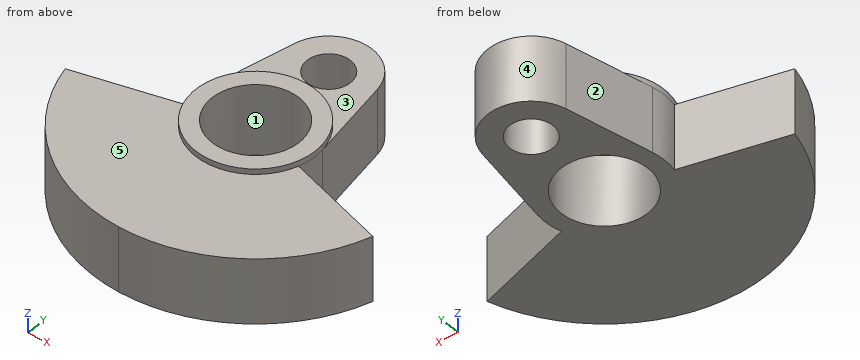
```python
from build123d import *
from build123d.topology import SkipClean

# Parameters (mm, degrees)
SKETCH1_R           = 2
SKETCH1_R_2         = 4
BOSS_EXTRUDE1_DEPTH = 6
BOSS_EXTRUDE2_START = -6
BOSS_EXTRUDE2_DEPTH = 6
SKETCH3_R           = 5.5
SKETCH3_R_2         = 4
BOSS_EXTRUDE4_DEPTH = 0.5


with BuildPart() as part:
    # Sketch1 → Boss-Extrude1 (new body)
    with BuildSketch(Plane.XY):
        with BuildLine():
            Line((-5.402455316, -6.96875), (-3.929058411, 0.75))
            ThreePointArc((-3.929058411, 0.75), (0, 4), (3.929058411, 0.75))
            Line((3.929058411, 0.75), (5.402455316, -6.96875))
            ThreePointArc((5.402455316, -6.96875), (0, -13.5), (-5.402455316, -6.96875))
        make_face()
        Circle(SKETCH1_R, mode=Mode.SUBTRACT)
        with Locations((0, -8)):
            Circle(SKETCH1_R_2, mode=Mode.SUBTRACT)
    extrude(amount=BOSS_EXTRUDE1_DEPTH)

    # Sketch2 → Boss-Extrude2 (add)
    with BuildSketch(Plane.XY.offset(6).offset(BOSS_EXTRUDE2_START)):
        with BuildLine():
            Line((0, -13.5), (0, -23))
            ThreePointArc((0, -23), (9.082951062, -19.937336386), (14.456832295, -12))
            Line((14.456832295, -12), (5.300838508, -9.466666667))
            ThreePointArc((5.300838508, -9.466666667), (3.33041539, -12.377023342), (0, -13.5))
        make_face()
        with BuildLine():
            Line((-5.300838508, -9.466666667), (-14.456832295, -12))
            ThreePointArc((-14.456832295, -12), (-9.082951062, -19.937336386), (0, -23))
            Line((0, -23), (0, -13.5))
            ThreePointArc((0, -13.5), (-3.33041539, -12.377023342), (-5.300838508, -9.466666667))
        make_face()
    extrude(amount=BOSS_EXTRUDE2_DEPTH)

    # Sketch3 → Boss-Extrude4 (add)
    with SkipClean():  # the faces are left unmerged after this step: merging them gives an invalid solid
        with BuildSketch(Plane.XY.offset(6)):
            with Locations(Location((0, -8, 0), (0, 0, 169.193077125))):
                Circle(SKETCH3_R)
            with Locations((0, -8)):
                Circle(SKETCH3_R_2, mode=Mode.SUBTRACT)
        extrude(amount=BOSS_EXTRUDE4_DEPTH)


solid = part.part
```
Verification items for the finished model (mm, model axes). Face numbers are marked on the shaded views. A direction names the side the tool comes from. Give positions to 0.01 mm unless a question says otherwise; leave off trailing zeros. Loops run counter-clockwise (first coordinate to the right, second up) from the corner with the lowest first, then second, coordinate; pieces in that order, holes last. Notation, with made-up numbers: M 82.5,-37.5 L 136.5,-37.5 A25 ccw 136.5,-8.5 Z; hole C 68,39.25 d1. An arc over 180 degrees is marked long. Return JSON: item names as keys, results as strings.
1) Mould release check, pull along Y, two halves, no side actions. Record for the marked faces 1, 2 and 3: released by +Y, released by -Y, zero draft, split by the parting line, or undercut.
Findings:
{"face 1": "undercut", "face 2": "released by +Y", "face 3": "zero draft"}
2) Gauge pin test, flat ends, axial feed: P1, Ø2, axis at y = -13.5, z = 1.5, coming from the -X side; P2, Ø3, axis at x = 2.5, z = 5.5, coming from the -Y side; P3, Ø5, axis at x = 0, y = -8, coming from the +Z side; P4, Ø10, axis at x = -10, y = -13.5, coming from the +Z side. Record the tip position at first contact, or that the pin passes through.
Findings:
{"P1": "stops at x = -14.31", "P2": "stops at y = -22.97", "P3": "passes through", "P4": "stops at z = 6"}
3) Tool access check on the marked faces 4 and 5. Record the directions out of +Z, -Z, +X, -X, +Y, -Y that give a thin tool (end or side, any length) a straight path to the whole face; none if there is none.
Findings:
{"face 4": "+Z, -Z, +Y", "face 5": "+Z, -Y"}
4) Section check D-D, the plane y = -5.25. Enter the section's corners in (x, z).
Findings:
{"outline": "M -5.07,0 L -2.9,0 L -2.9,6.5 L -4.76,6.5 L -4.76,6 L -5.07,6 Z; M 2.9,0 L 5.07,0 L 5.07,6 L 4.76,6 L 4.76,6.5 L 2.9,6.5 Z"}
5) Section check C-C, the plane z = 1. Enter the section's corners in (x, y), and give its area (4 significant figures).
Findings:
{"outline": "M -14.46,-12 A15 ccw 14.46,-12 L 5.3,-9.47 A5.5 ccw 5.4,-6.97 L 3.93,0.75 A4 ccw -3.93,0.75 L -5.4,-6.97 A5.5 ccw -5.3,-9.47 Z; hole C 0,-8 d8; hole C 0,0 d4", "area": "340.5 mm2"}
6) Section check A-A, the plane y = -8. Enter the section's corners in (x, z), and give its area (3 significant figures).
Findings:
{"outline": "M -5.5,0 L -4,0 L -4,6.5 L -5.5,6.5 Z; M 4,0 L 5.5,0 L 5.5,6.5 L 4,6.5 Z", "area": "19.5 mm2"}
7) Section check B-B, the plane x = -2.5. Enter the section's corners in (y, z), and give its area (3 significant figures).
Findings:
{"outline": "M -22.79,0 L -11.12,0 L -11.12,6.5 L -12.9,6.5 L -12.9,6 L -22.79,6 Z; M -4.88,0 L 3.12,0 L 3.12,6 L -3.1,6 L -3.1,6.5 L -4.88,6.5 Z", "area": "120 mm2"}
8) Material ranges on L1, parallel to Y at x = 1.5, z = 4.25; L2, parallel to Y at x = -3.5, z = 0.5; L3, parallel to Y at x = -2.25, z = 2.5, recorded low to high. Write a range as [from, to].
Findings:
{"L1": "y = [-22.92, -11.71], [-4.29, -1.32], [1.32, 3.71]", "L2": "y = [-22.59, -9.94], [-6.06, 1.94]", "L3": "y = [-22.83, -11.31], [-4.69, 3.31]"}
